Could you check a few things on this model? Use its own coordinates, in mm. A direction names the side the tool comes from. Give positions to 0.01 mm unless a question says otherwise; leave off trailing zeros. Order: outer loops, then holes, each group sorted by start corner. A loop starts at its lowest first (then second) coordinate and runs counter-clockwise, first axis right, second up. Notation, with made-up numbers: (-35, 72.25) -> (-14, 72.25) arc R25 ccw to (-14, 85.25) -> close; hole circle Ø5 at (-7, -24). An arc over 180 degrees is marked (long way). Answer as CSV lines item,"result". Start each with the question number.
(1) Will these pins go through, and if not, where does the flat tip stop? pin 1 Ø1.5 at (x, z) = (11.5, -5.5) entering from +Y; pin 2 Ø16 at (x, z) = (8.5, -16.5) entering from +Y; pin 3 Ø4 at (x, z) = (20, -26) entering from +Y; pin 4 Ø1.8 at (x, z) = (-20, -26) entering from -Y.
(2) I want a section at C-C (z = -3). Please give me the cut outline in (x, y).
(3) I want a section at A-A (y = 18.5). Please give me the cut outline in (x, z), plus the area to 3 significant figures.
(4) On a 3-axis mill with a long thin cutter (end or side, diameter ignored), from which of +Z, -Z, +X, -X, +Y, -Y can I reach the whole of each face in a straight line? I mean faces 1 (the face through (-24, -3, -17)), 2 (the face through (6.386, -12.925, -5.07)). Say none if no direction works.
(5) I want a section at D-D (y = -1.5). Please give me the cut outline in (x, z), plus the area to 3 significant figures.
(6) I want a section at B-B (x = 0). Please give me the cut outline in (y, z), plus the area to 3 significant figures.
(7) We'd pull the mould along Z, two halves only. Please class faces 3 (the face through (-21.664, 33.324, -14.936)), 4 (the face through (21.01, -18.48, -15.11)), 5 (the face through (-25, 0, -1)), 6 (the face through (0, -10, -6)): released by +Z, released by -Z, zero draft, split by the parting line, or undercut.
(8) I need wall thicknesses on L1, parallel to X at y = -19.1, z = -14; L2, parallel to X at y = 1, z = -13; L3, parallel to X at y = -18.6, z = -26. Which ranges of each line are inside material? Lowest first, please.
```python
from build123d import *

# Parameters (mm, degrees)
BOSS_EXTRUDE1_DEPTH     = 30
SKETCH3_4_R             = 10
BOSS_EXTRUDE2_DEPTH     = 10
CUT_EXTRUDE2_DEPTH      = 62.951594007
CUT_EXTRUDE2_DEPTH_BACK = 62.951594007
CUT_EXTRUDE3_START      = -8
SKETCH6_W               = 22
SKETCH6_H               = 41
SKETCH6_R               = 10
CUT_EXTRUDE3_DEPTH      = 8
SKETCH6_3_R             = 1.5
CUT_EXTRUDE4_DEPTH      = 58.775427431
CUT_EXTRUDE5_DEPTH      = 79.217645188
SKETCH8_R               = 1.5
CUT_EXTRUDE6_DEPTH      = 76.663729872
FILLET1_R               = 5


with BuildPart() as part:
    # Sketch3 → Boss-Extrude1 (new body)
    with BuildSketch(Plane.XY):
        with BuildLine():
            ThreePointArc((-27, 20), (0, 47), (27, 20))
            Line((27, 20), (27, -20))
            Line((27, -20), (-27, -20))
            Line((-27, -20), (-27, 20))
        make_face()
        with BuildLine():
            Line((-24, -17), (-24, 20))
            ThreePointArc((-24, 20), (0, 44), (24, 20))
            Line((24, 20), (24, -17))
            Line((24, -17), (-24, -17))
        make_face(mode=Mode.SUBTRACT)
    extrude(amount=-BOSS_EXTRUDE1_DEPTH)

    # Sketch3_4 → Boss-Extrude2 (add)
    with BuildSketch(Plane.XY):
        with BuildLine():
            ThreePointArc((-24, 20), (0, 44), (24, 20))
            Line((24, 20), (24, -17))
            Line((24, -17), (-24, -17))
            Line((-24, -17), (-24, 20))
        make_face()
        with Locations((0, 20)):
            Circle(SKETCH3_4_R, mode=Mode.SUBTRACT)
    extrude(amount=-BOSS_EXTRUDE2_DEPTH)

    # Sketch5 → Cut-Extrude2 (cut, two sides: drawn at the far end of the back side and taken through both)
    with BuildSketch(Plane(origin=(0, 0, 0), x_dir=(0, 0, -1), z_dir=(1, 0, 0)).offset(-CUT_EXTRUDE2_DEPTH_BACK)):
        with BuildLine():
            Line((15.255034443, 32.183889783), (30, -15))
            Line((30, -15), (30, 47))
            Line((30, 47), (15, 47))
            ThreePointArc((15, 47), (14.181044165, 40.740478791), (14.690093427, 34.448168938))
            ThreePointArc((14.690093427, 34.448168938), (14.93950997, 33.307782347), (15.255034443, 32.183889783))
        make_face()
    extrude(amount=CUT_EXTRUDE2_DEPTH + CUT_EXTRUDE2_DEPTH_BACK, mode=Mode.SUBTRACT)

    # Sketch6 → Cut-Extrude3 (cut)
    with BuildSketch(Plane(origin=(0, 0, -10), x_dir=(-1, 0, 0), z_dir=(0, 0, -1)).offset(CUT_EXTRUDE3_START)):
        with Locations((0, 10.5)):
            Rectangle(SKETCH6_W, SKETCH6_H)
        with Locations(Location((0, 20, 0), (0, 0, 180))):
            Circle(SKETCH6_R, mode=Mode.SUBTRACT)
    extrude(amount=CUT_EXTRUDE3_DEPTH, mode=Mode.SUBTRACT)

    # Sketch6_3 → Cut-Extrude4 (cut, through all)
    with BuildSketch(Plane(origin=(0, 0, -10), x_dir=(-1, 0, 0), z_dir=(0, 0, -1))):
        with Locations((-5, 34.5)):
            Circle(SKETCH6_3_R)
        with Locations((5, 34.5)):
            Circle(SKETCH6_3_R)
        with Locations(Location((5, -13.5, 0), (0, 0, 180))):
            Circle(SKETCH6_3_R)
        with Locations(Location((-5, -13.5, 0), (0, 0, 180))):
            Circle(SKETCH6_3_R)
    extrude(amount=-CUT_EXTRUDE4_DEPTH, mode=Mode.SUBTRACT)

    # Sketch7 → Cut-Extrude5 (cut, through all)
    with BuildSketch(Plane.XZ.offset(20)):
        with BuildLine():
            Line((-27, -25), (-27, -30))
            Line((-27, -30), (-22, -30))
            ThreePointArc((-22, -30), (-25.535533906, -28.535533906), (-27, -25))
        make_face()
        with BuildLine():
            Line((22, -30), (27, -30))
            Line((27, -30), (27, -25))
            ThreePointArc((27, -25), (25.535533906, -28.535533906), (22, -30))
        make_face()
    extrude(amount=-CUT_EXTRUDE5_DEPTH, mode=Mode.SUBTRACT)

    # Sketch8 → Cut-Extrude6 (cut, through all)
    with BuildSketch(Plane(origin=(0, -17, 0), x_dir=(1, 0, 0), z_dir=(0, 1, 0))):
        with Locations(Location((-20, 26, 0), (0, 0, 270))):
            Circle(SKETCH8_R)
        with Locations(Location((20, 26, 0), (0, 0, 270))):
            Circle(SKETCH8_R)
        with Locations(Location((20, 14, 0), (0, 0, 270))):
            Circle(SKETCH8_R)
        with Locations(Location((-20, 14, 0), (0, 0, 270))):
            Circle(SKETCH8_R)
    extrude(amount=-CUT_EXTRUDE6_DEPTH, mode=Mode.SUBTRACT)

    # Fillet1
    fillet1_edges = [part.edges().sort_by_distance(p)[0] for p in [
        (27, 0, 0),
        (-27, 0, 0),
        (0, 47, 0),
    ]]
    fillet(fillet1_edges, radius=FILLET1_R)


solid = part.part
```
Final values:
1,pin 1,"y = 44.77"
1,pin 2,"y = 46.99"
1,pin 3,"y = -17"
1,pin 4,"through"
2,outline,"(-26.58, -20) -> (26.58, -20) -> (26.58, 20) arc R26.58 ccw to (-26.58, 20) -> close; hole (-11, -10) -> (11, -10) -> (11, 31) -> (-11, 31) -> close; hole circle Ø3 at (-5, -13.5); hole circle Ø3 at (-5, 34.5); hole circle Ø3 at (5, -13.5); hole circle Ø3 at (5, 34.5)"
3,outline,"(-27, -19.53) -> (-24, -19.53) -> (-24, -10) -> (-11, -10) -> (-11, -2) -> (-9.89, -2) -> (-9.89, 0) -> (-22, 0) arc R5 ccw to (-27, -5) -> close; (9.89, -2) -> (11, -2) -> (11, -10) -> (24, -10) -> (24, -19.53) -> (27, -19.53) -> (27, -5) arc R5 ccw to (22, 0) -> (9.89, 0) -> close"
3,area,"371 mm²"
4,face 1,"-Z"
4,face 2,"+Z, -Z"
5,outline,"(-27, -25) arc R5 ccw to (-26.94, -25.78) -> (-24, -25.78) -> (-24, -10) -> (-11, -10) -> (-11, -2) -> (11, -2) -> (11, -10) -> (24, -10) -> (24, -25.78) -> (26.94, -25.78) arc R5 ccw to (27, -25) -> (27, -5) arc R5 ccw to (22, 0) -> (-22, 0) arc R5 ccw to (-27, -5) -> close"
5,area,"448 mm²"
6,outline,"(-20, -30) -> (-17, -30) -> (-17, -10) -> (-10, -10) -> (-10, -2) -> (10, -2) -> (10, 0) -> (-20, 0) -> close; (30, -2) -> (31, -2) -> (31, -10) -> (44, -10) -> (44, -14.44) arc R30 cw to (47, -15) -> (47, -5) arc R5 ccw to (42, 0) -> (30, 0) -> close"
6,area,"371 mm²"
7,face 3,"released by -Z"
7,face 4,"undercut"
7,face 5,"released by +Z"
7,face 6,"zero draft"
8,L1,"-27 to -21.5, -18.5 to 18.5, 21.5 to 27"
8,L2,"-27 to -24, 24 to 27"
8,L3,"-26.9 to -21.5, -18.5 to 18.5, 21.5 to 26.9"
